from build123d import *

# Parameters (mm, degrees)
SKETCH1_R           = 4.7625
BOSS_EXTRUDE1_DEPTH = 6.35


with BuildPart() as part:
    # Sketch1 → Boss-Extrude1 (new body)
    with BuildSketch(Plane(origin=(0, 0, 0), x_dir=(0, 0, -1), z_dir=(1, 0, 0))):
        with BuildLine():
            Line((-16.51, -19.05), (-10.4267, -19.05))
            Line((-10.4267, -19.05), (-10.4267, -16.51))
            ThreePointArc((-10.4267, -16.51), (-9.682751224, -14.713948776), (-7.8867, -13.97))
            Line((-7.8867, -13.97), (7.8867, -13.97))
            ThreePointArc((7.8867, -13.97), (9.682751224, -14.713948776), (10.4267, -16.51))
            Line((10.4267, -16.51), (10.4267, -19.05))
            Line((10.4267, -19.05), (16.51, -19.05))
            Line((16.51, -19.05), (16.51, -8.89))
            Line((16.51, -8.89), (12.9667, -8.89))
            ThreePointArc((12.9667, -8.89), (11.170648776, -8.146051224), (10.4267, -6.35))
            Line((10.4267, -6.35), (10.4267, 0))
            ThreePointArc((10.4267, 0), (0, 10.4267), (-10.4267, 0))
            Line((-10.4267, 0), (-10.4267, -6.35))
            ThreePointArc((-10.4267, -6.35), (-11.170648776, -8.146051224), (-12.9667, -8.89))
            Line((-12.9667, -8.89), (-16.51, -8.89))
            Line((-16.51, -8.89), (-16.51, -19.05))
        make_face()
        with Locations(Location((0, 0, 0), (0, 0, 180))):
            Circle(SKETCH1_R, mode=Mode.SUBTRACT)
    extrude(amount=BOSS_EXTRUDE1_DEPTH)


solid = part.part
Read the model definition and answer for the solid it produces. Units are mm, in the model's axes. A direction names the side the tool comes from. Coordinates: 2 decimals unless noted, no trailing zeros. Order: outer loops, then holes, each group sorted by start corner. A loop starts at its lowest first (then second) coordinate and runs counter-clockwise, first axis right, second up. Notation, with made-up numbers: (-11, 28.5) - (1, 28.5) arc R23 ccw to (1, 64.5) - close; hole circle Ø9 at (6.25, 8.5). An arc over 180 degrees is marked (long way). Use one line per item in the form item = value.
(1) Straight lines are drawn through the part: L1, parallel to Y at x = 3.25, z = 0; L2, parallel to Z at x = 5.5, y = -16.75; L3, parallel to Y at x = 5.25, z = 2. For each, find the intervals that lie inside material, in ascending order.
Computed values:
L1 = -13.97 to -4.76, 4.76 to 10.43
L2 = -16.51 to -10.43, 10.43 to 16.51
L3 = -13.97 to -4.32, 4.32 to 10.23
(2) Section A-A, the plane z = 0 is taken. Give the vertices of the cut face in (x, y).
Computed values:
outline = (0, -13.97) - (6.35, -13.97) - (6.35, -4.76) - (0, -4.76) - close; (0, 4.76) - (6.35, 4.76) - (6.35, 10.43) - (0, 10.43) - close
(3) Section D-D, the plane z = 14 is taken. Give the vertices of the cut face in (x, y), then the cut area to 3 significant figures.
Computed values:
outline = (0, -19.05) - (6.35, -19.05) - (6.35, -8.89) - (0, -8.89) - close
area = 64.5 mm²
(4) Given pin 1 Ø3 at (x, z) = (3.5, 3.5) entering from -Y; pin 2 Ø2 at (x, y) = (3, 0.5) entering from -Z; pin 3 Ø1.1 at (x, z) = (2, -14.5) entering from +Y; pin 4 Ø8.5 at (y, z) = (0, 0) entering from -X, each flat-ended and moving along its own axis, determine where each tip first touches the part or whether it passes through.
Computed values:
pin_1 = -13.97
pin_2 = -10.43
pin_3 = -8.89
pin_4 = through
(5) Section B-B, the plane y = -2 is taken. Give the vertices of the cut face in (x, z).
Computed values:
outline = (0, -10.43) - (6.35, -10.43) - (6.35, -4.32) - (0, -4.32) - close; (0, 4.32) - (6.35, 4.32) - (6.35, 10.43) - (0, 10.43) - close
(6) Which of the six approach directions +Z, -Z, +X, -X, +Y, -Y give full straight-line access (tool end or side, diameter ignored) to faces 4 (the face through (3, -3, -10.427)), 5 (the face through (3.13, -14.69, -9.66)), 6 (the face through (3, -3, 10.427))?
Computed values:
face_4 = -Z, +X, -X, +Y
face_5 = +X, -X, -Y
face_6 = +Z, +X, -X, +Y
(7) For a pull along Z with two mould halves and no side action, classify faces 1 (the face through (3, -19.05, -13)), 2 (the face through (3.13, 4.65, -1.03)), 3 (the face through (3.131, -8.166, -11.191)) as pulls with the +Z half, pulls with the -Z half, needs draft (parallel to the pull), parting line crosses it, or undercut.
Computed values:
face_1 = needs draft
face_2 = undercut
face_3 = pulls with the -Z half
